from build123d import *

# Parameters (mm, degrees)
SKETCH1_W           = 74
SKETCH1_H           = 96
BOSS_EXTRUDE1_DEPTH = 45
SKETCH2_W           = 68
SKETCH2_H           = 90
CUT_EXTRUDE1_DEPTH  = 40
SKETCH3_R           = 3
SKETCH3_R_2         = 5
CUT_EXTRUDE2_DEPTH  = 40
FILLET1_R           = 3


with BuildPart() as part:
    # Sketch1 → Boss-Extrude1 (new body)
    with BuildSketch(Plane(origin=(0, 0, 0), x_dir=(1, 0, 0), z_dir=(0, 1, 0))):
        with Locations((37, -48)):
            Rectangle(SKETCH1_W, SKETCH1_H)
    extrude(amount=BOSS_EXTRUDE1_DEPTH)

    # Sketch2 → Cut-Extrude1 (cut)
    with BuildSketch(Plane(origin=(0, 45, 0), x_dir=(1, 0, 0), z_dir=(0, 1, 0))):
        with Locations((37, -48)):
            Rectangle(SKETCH2_W, SKETCH2_H)
    extrude(amount=-CUT_EXTRUDE1_DEPTH, mode=Mode.SUBTRACT)

    # Sketch3 → Cut-Extrude2 (cut)
    with BuildSketch(Plane.XZ):
        with Locations((24, 81.8)):
            Circle(SKETCH3_R)
        with Locations((37, 60)):
            Circle(SKETCH3_R_2)
    extrude(amount=-CUT_EXTRUDE2_DEPTH, mode=Mode.SUBTRACT)

    # Fillet1
    fillet1_edges = [part.edges().sort_by_distance(p)[0] for p in [
        (37, 0, 0),
        (74, 0, 48),
        (37, 0, 96),
        (0, 0, 48),
        (0, 22.5, 0),
        (74, 22.5, 0),
        (74, 22.5, 96),
        (0, 22.5, 96),
    ]]
    fillet(fillet1_edges, radius=FILLET1_R)


solid = part.part
Design review of the part built by this model. Coordinates are the model's own, in mm. A direction names the side the tool comes from. Coordinates: 2 decimals unless noted, no trailing zeros. Loops run counter-clockwise (first coordinate to the right, second up) from the corner with the lowest first, then second, coordinate; pieces in that order, holes last. Notation, with made-up numbers: M 48,74.5 L 92,74.5 A22 cw 92,99.5 Z; hole C 71,28.25 d6. An arc over 180 degrees is marked long. Answer as CSV lines item,"result".
Item 1: Machinability: for faces 1 (the face through (37, 5, 47)), 2 (the face through (0.86, 24.29, 0.9)), which of the approach directions +Z, -Z, +X, -X, +Y, -Y give a long, thin tool a straight path to every point of the face, cutting with its end or side? Answer none if there is none.
Answer list:
face 1,"+Y"
face 2,"-Z, -X, +Y, -Y"
Item 2: Add section C-C on y = 18. State the section outline as (x, z) points, plus the area to 3 significant figures.
Answer list:
outline,"M 0,3 A3 ccw 3,0 L 71,0 A3 ccw 74,3 L 74,93 A3 ccw 71,96 L 3,96 A3 ccw 0,93 Z; hole M 3,3 L 71,3 L 71,93 L 3,93 Z"
area,"976 mm²"
Item 3: Add section B-B on x = 24. State the section outline as (y, z) points, plus the area to 3 significant figures.
Answer list:
outline,"M 0,3 A3 ccw 3,0 L 45,0 L 45,3 L 5,3 L 5,78.8 L 0,78.8 Z; M 0,84.8 L 5,84.8 L 5,93 L 45,93 L 45,96 L 3,96 A3 ccw 0,93 Z"
area,"686 mm²"
Item 4: Add section D-D on x = 65. State the section outline as (y, z) points, plus the area to 3 significant figures.
Answer list:
outline,"M 0,3 A3 ccw 3,0 L 45,0 L 45,3 L 5,3 L 5,93 L 45,93 L 45,96 L 3,96 A3 ccw 0,93 Z"
area,"716 mm²"
Item 5: For probe 1 along Z at (x, y) = (51, 18); probe 2 along X at (y, z) = (22, 77); probe 3 along Z at (x, y) = (37, 2.7), list the stretches that pass through material, from the lowest coordinate up.
Answer list:
probe 1,"0 to 3, 93 to 96"
probe 2,"0 to 3, 71 to 74"
probe 3,"0.02 to 55, 65 to 95.98"
Item 6: Add section A-A on z = 81.8. State the section outline as (x, y) points.
Answer list:
outline,"M 0,3 A3 ccw 3,0 L 21,0 L 21,5 L 3,5 L 3,45 L 0,45 Z; M 27,0 L 71,0 A3 ccw 74,3 L 74,45 L 71,45 L 71,5 L 27,5 Z"
Item 7: The part is to be moulded in two halves that separate along X. For faces 3 (the face through (0, 24, 49)), 4 (the face through (73.1, 24.29, 95.14)), 5 (the face through (21.6, 2.5, 80)), 6 (the face through (37, 0, 47)), say which applies: pulls with the +X half, pulls with the -X half, needs draft (parallel to the pull), parting line crosses it, or undercut.
Answer list:
face 3,"pulls with the -X half"
face 4,"pulls with the +X half"
face 5,"undercut"
face 6,"needs draft"
